from build123d import *

# Parameters (mm, degrees)
BOSS_EXTRUDE1_DEPTH = 0.8
CHAMFER1_SIZE       = 1.2
CHAMFER1_SIZE_2     = 0.8
CUT_EXTRUDE1_REACH  = 26.533
SKETCH5_R           = 1.4


with BuildPart() as part:
    # Sketch2 → Boss-Extrude1 (new body)
    with BuildSketch(Plane.XY):
        with BuildLine():
            Line((-7, 0), (-0.3, 0))
            Line((-0.3, 0), (-0.3, 20))
            Line((-0.3, 20), (-0.3, 21.417744688))
            ThreePointArc((-0.3, 21.417744688), (-4.224568837, 23.424178734), (-7, 20))
            Line((-7, 20), (-7, 0))
        make_face()
    extrude(amount=BOSS_EXTRUDE1_DEPTH)

    # Chamfer1
    # the kernel refuses this chamfer: 1.2, 0.8 mm, written as the material it takes off along each edge
    with BuildSketch(Plane(origin=(-0.3, 24.518305317, 0.8), x_dir=(-0.9997695277037822, 0, 0.021468383147227363), z_dir=(0, -1, 0))) as chamfer1_piece_1:
        Polygon((CHAMFER1_SIZE * 0.999769527704, CHAMFER1_SIZE * 0.0214683831472), (-CHAMFER1_SIZE_2 * 0.0214683831472, CHAMFER1_SIZE_2 * 0.999769527704), (0, 0), align=None)
    extrude(amount=27.618865945, mode=Mode.SUBTRACT)

    # Sketch5 → Cut-Extrude1 (cut, up to next)
    with BuildSketch(Plane.XY.offset(0.8), mode=Mode.PRIVATE) as cut_extrude1_sk1:
        with Locations((-4.3, 11.4)):
            Circle(SKETCH5_R)
    cut_extrude1_tool1 = extrude(cut_extrude1_sk1.sketch, amount=-CUT_EXTRUDE1_REACH, mode=Mode.PRIVATE) & part.part
    add(cut_extrude1_tool1.solids().sort_by_distance((-4.3, 11.4, 0.8))[0], mode=Mode.SUBTRACT)


solid = part.part
Check sheet for the modelled part. Datum: model origin and axes. Units: mm. Give positions to 0.01 mm unless a question says otherwise; leave off trailing zeros. Order: outer loops, then holes, each group sorted by start corner. A loop starts at its lowest first (then second) coordinate and runs counter-clockwise, first axis right, second up. Notation, with made-up numbers: M -30.75,57 L -9.75,57 A23 cw -9.75,87 Z; hole C 22,75 d5. An arc over 180 degrees is marked long. Answer as CSV lines item,"result". Start each with the question number.
Item 1: Cross-section at D-D on y = 5.5. Enter the section's corners in (x, z), plus the area to 3 significant figures.
Item 2: Cross-section at B-B on x = -4. Enter the section's corners in (y, z), plus the area to 3 significant figures.
Item 3: Thickness scan on line 1 (Y direction, x = -3.25, z = 0.55); line 2 (Y direction, x = -4.3, z = 0.4); line 3 (X direction, y = 12.5, z = 0.4). Record the ranges inside material, lowest first. Write a range as [from, to].
Item 4: Cross-section at C-C on z = 0.5. Enter the section's corners in (x, y), plus the area to 3 significant figures.
Item 5: Mould release check, pull along Y, two halves, no side actions. Record for faces 1 (the face through (-2, 12, 0)), 2 (the face through (-2.965, 11.821, 0.406)), 3 (the face through (-4.159, 23.437, 0.394)): +Y half, -Y half, draft (parallel to the pull), parting line (faces both ways), or undercut.
Item 6: Cross-section at A-A on y = 11.4. Enter the section's corners in (x, z).
Established:
1,outline,"M -7,0 L -0.3,0 L -1.5,0.8 L -7,0.8 Z"
1,area,"4.88 mm^2"
2,outline,"M 0,0 L 10.03,0 L 10.03,0.8 L 0,0.8 Z; M 12.77,0 L 23.46,0 L 23.46,0.8 L 12.77,0.8 Z"
2,area,"16.6 mm^2"
3,line 1,"y = [0, 10.47], [12.33, 23.49]"
3,line 2,"y = [0, 10], [12.8, 23.41]"
3,line 3,"x = [-7, -5.17], [-3.43, -0.9]"
4,outline,"M -7,0 L -1.05,0 L -1.05,22.5 A3.5 ccw -7,20 Z; hole C -4.3,11.4 d2.8"
4,area,"130 mm^2"
5,face 1,"draft"
5,face 2,"undercut"
5,face 3,"+Y half"
6,outline,"M -7,0 L -5.7,0 L -5.7,0.8 L -7,0.8 Z; M -2.9,0 L -0.3,0 L -1.5,0.8 L -2.9,0.8 Z"
